For this review, take the finished solid that the model builds, in its own axes (mm). Face numbers are marked on the shaded views. A direction names the side the tool comes from. Round coordinates to 2 decimals unless told otherwise and drop trailing zeros. Loops run counter-clockwise (first coordinate to the right, second up) from the corner with the lowest first, then second, coordinate; pieces in that order, holes last. Notation, with made-up numbers: (12, 45) -> (31, 45) arc R5 cw to (31, 49) -> close; hole circle Ø5 at (-32.75, 65). An arc over 180 degrees is marked (long way). One line per question, with ' | ' between items. Start each with the question number.
1. Draft analysis for pull direction X (two halves, no side actions). For the marked faces 4, 5 and 6, state which applies: pulls with the +X half, pulls with the -X half, needs draft (parallel to the pull), parting line crosses it, or undercut.
2. Consider section A-A (x = 234). Write out the cut boundary in (y, z), and give its area (3 significant figures).
3. Consider section D-D (y = -3.5). Write out the cut boundary in (x, z).
4. Consider section B-B (z = -9.63). Write out the cut boundary in (x, y), and give its area (3 significant figures).
5. Wall thickness on line 1 along Z through (x, y) = (222.5, -1.5); line 2 along Z through (x, y) = (239, -8.25); line 3 along Y through (x, z) = (246, -6): over which ranges is each line inside the solid? List them lowest first.
6. For the marked faces 1, 2 and 3, list the 3-axis set-ups (+Z, -Z, +X, -X, +Y, -Y) from which the entire face can be reached by the end or side of a thin tool; tool diameter is ignored.
7. For pin 1 Ø3 at (x, z) = (234.5, -10.5) entering from -Y; pin 2 Ø6 at (x, y) = (235.5, -2) entering from -Z; pin 3 Ø2 at (x, y) = (238.5, 1.5) entering from -Z, all flat-tipped, find the tip position at first contact; note any pin that passes through.
8. Consider section C-C (x = 239). Write out the cut boundary in (y, z), and give its area (3 significant figures).
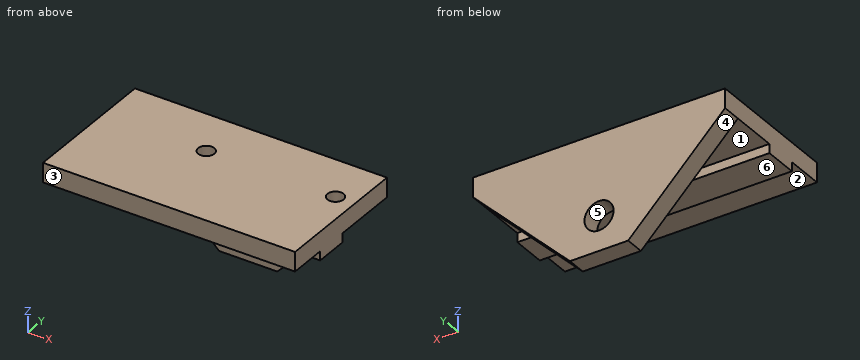
```python
from build123d import *

# Parameters (mm, degrees)
ESQUISSE1_W                                   = 39
ESQUISSE1_H                                   = 18.5
BOSS_EXTRU_1_DEPTH                            = 3
ESQUISSE4_W                                   = 1.4
ESQUISSE4_H                                   = 5.26
BOSS_EXTRU_2_DEPTH                            = 39
TROU_POUR_TARAUDAGE_POUR_TROU_TARAUD_M3_D     = 2.5
TROU_POUR_TARAUDAGE_POUR_TROU_TARAUD_M3_DEPTH = 16
ESQUISSE7_W                                   = 39
ESQUISSE7_H                                   = 18
BOSS_EXTRU_3_DEPTH                            = 3
CHANFREIN1_SIZE                               = 15
D_GAGEMENT_M42_D                              = 4.5
D_GAGEMENT_M42_DEPTH                          = 16


with BuildPart() as part:
    # Esquisse1 → Boss.-Extru.1 (new body)
    with BuildSketch(Plane.XY):
        with Locations((235.738481082, -2.221059771)):
            Rectangle(ESQUISSE1_W, ESQUISSE1_H)
    extrude(amount=BOSS_EXTRU_1_DEPTH)

    # Esquisse4 → Boss.-Extru.2 (add)
    with BuildSketch(Plane(origin=(255.238481082, 0, 0), x_dir=(0, 0, -1), z_dir=(1, 0, 0))):
        with Locations((0.7, -2.971059771)):
            Rectangle(ESQUISSE4_W, ESQUISSE4_H)
    extrude(amount=-BOSS_EXTRU_2_DEPTH)

    # Trou pour taraudage pour trou taraudé M31
    with Locations(Plane.XY.offset(3)):
        with Locations((232.238481082, 2.528940229), (252.238481082, 2.528940229)):
            Hole(TROU_POUR_TARAUDAGE_POUR_TROU_TARAUD_M3_D / 2, depth=TROU_POUR_TARAUDAGE_POUR_TROU_TARAUD_M3_DEPTH)

    # Esquisse7 → Boss.-Extru.3 (add)
    with BuildSketch(Plane(origin=(0, 7.028940229, 0), x_dir=(1, 0, 0), z_dir=(0, 1, 0))):
        with Locations((235.738481082, 6)):
            Rectangle(ESQUISSE7_W, ESQUISSE7_H)
    extrude(amount=BOSS_EXTRU_3_DEPTH)

    # Chanfrein1
    chanfrein1_edges = [part.edges().sort_by_distance(p)[0] for p in [
        (216.238481082, 8.528940229, -15),
        (255.238481082, 8.528940229, -15),
    ]]
    chamfer(chanfrein1_edges, length=CHANFREIN1_SIZE)

    # Dégagement M42
    with Locations(Plane(origin=(0, 10.028940229, 0), x_dir=(1, 0, 0), z_dir=(0, 1, 0))):
        with Locations((235.738481082, 9.63)):
            Hole(D_GAGEMENT_M42_D / 2, depth=D_GAGEMENT_M42_DEPTH)


solid = part.part
```
Answer block:
1) face 4: pulls with the -X half | face 5: undercut | face 6: needs draft
2) outline: (-11.47, 0) -> (-5.6, 0) -> (-5.6, -1.4) -> (-0.34, -1.4) -> (-0.34, 0) -> (7.03, 0) -> (7.03, -8.2) -> (10.03, -8.2) -> (10.03, 3) -> (-11.47, 3) -> close; (7.03, -15) -> (10.03, -15) -> (10.03, -11.06) -> (7.03, -11.06) -> close | area: 108 mm2
3) outline: (216.24, -1.4) -> (255.24, -1.4) -> (255.24, 3) -> (216.24, 3) -> close
4) outline: (225.87, 7.03) -> (233.49, 7.03) -> (233.49, 10.03) -> (225.87, 10.03) -> close; (237.99, 7.03) -> (245.61, 7.03) -> (245.61, 10.03) -> (237.99, 10.03) -> close | area: 45.7 mm2
5) line 1: z = -1.4 to 3 | line 2: z = 0 to 3 | line 3: y = 7.03 to 10.03
6) face 1: -Z, +X, -X | face 2: -Z, +X, -X, -Y | face 3: +Z, -Z, +X, -X, -Y
7) pin 1: stops at y = 7.03 | pin 2: stops at z = -1.4 | pin 3: stops at z = 0
8) outline: (-11.47, 0) -> (-5.6, 0) -> (-5.6, -1.4) -> (-0.34, -1.4) -> (-0.34, 0) -> (7.03, 0) -> (7.03, -15) -> (10.03, -15) -> (10.03, 3) -> (-11.47, 3) -> close | area: 117 mm2
